For this review, take the finished solid that the model builds, in its own axes (mm). A direction names the side the tool comes from. Round coordinates to 2 decimals unless told otherwise and drop trailing zeros. Order: outer loops, then holes, each group sorted by start corner. A loop starts at its lowest first (then second) coordinate and runs counter-clockwise, first axis right, second up. Notation, with made-up numbers: (-25.5, 5) -> (-12.5, 5) arc R12 cw to (-12.5, 19) -> close; hole circle Ø7 at (24, 32.5). An arc over 180 degrees is marked (long way). Use a Markdown table: item, result. Add a question column.
1) Consider section D-D (x = 38). State the section outline as (y, z) points (3 decimals).
2) Consider section C-C (z = -15). State the section outline as (x, y) points.
3) Consider section A-A (z = -29). State the section outline as (x, y) points.
4) Consider section B-B (y = 17). State the section outline as (x, z) points (3 decimals), plus the area to 3 significant figures.
5) Machinability: for faces 1 (the face through (119.412, 9.536, -0.028)), 2 (the face through (-119, 4, -6.35)), 3 (the face through (-51.782, 9.658, -12.017)), which of the approach directions +Z, -Z, +X, -X, +Y, -Y give a long, thin tool a straight path to every point of the face, cutting with its end or side? Answer none if there is none.
6) Draft analysis for pull direction Z (two halves, no side actions). For faces 4 (the face through (1, 9, 0)), 5 (the face through (1, 0, -6)), 6 (the face through (-118.87, 10.03, -4.92)), 7 (the face through (5, 9, -9.525)), state which applies: pulls with the +Z half, pulls with the -Z half, needs draft (parallel to the pull), parting line crosses it, or undercut.
7) Clearance check with flat-ended pins moving along their axes: P1, Ø4, axis at y = 5, z = -19, coming from the -X side; P2, Ø8, axis at x = 121, y = 4, coming from the +Z side; P3, Ø1, axis at y = 16.5, z = -14.5, coming from the -X side. State where each tip first meets the part, or that it passes through.
8) Wall thickness on line 1 along X through (y, z) = (16, -1); line 2 along Y through (x, z) = (31.75, -6) (3 decimals); line 3 along X through (y, z) = (6.5, -20): over which ranges is each line inside the solid? List them lowest first. Write a range as [from, to].
```python
from build123d import *

# Parameters (mm, degrees)
BOSS_EXTRUDE1_DEPTH            = 19.05
FILLET1_R                      = 19.05
SKETCH2_R                      = 1.5
CUT_EXTRUDE1_DEPTH             = 129.572996096
BOSS_EXTRUDE2_REACH            = 132.835
BOSS_EXTRUDE2_END_RADIUS       = 25.4
CUT_EXTRUDE3_REACH             = 132.835
CUT_EXTRUDE3_DIRECTION_2_DEPTH = 131.83465787
CUT_EXTRUDE2_DEPTH             = 131.83465787
CUT_EXTRUDE2_DEPTH_BACK        = 131.83465787
FILLET2_R                      = 3.175
FILLET2_OF_MIRROR1_R           = 3.175
CUT_EXTRUDE4_DEPTH             = 131.834658007
CUT_EXTRUDE4_DEPTH_BACK        = 131.834658007


with BuildPart() as part:
    # Sketch1 → Boss-Extrude1 (new body)
    with BuildSketch(Plane(origin=(0, 0, 0), x_dir=(1, 0, 0), z_dir=(0, 1, 0))):
        with BuildLine():
            ThreePointArc((-54.639410761, 9.525), (-93.706612459, 35.233649778), (-124.46, 0))
            Line((-124.46, 0), (-114.3, 0))
            ThreePointArc((-114.3, 0), (-88.9, 25.4), (-63.5, 0))
            Line((-63.5, 0), (-53.34, 0))
            ThreePointArc((-53.34, 0), (-53.666350222, 4.806612459), (-54.639410761, 9.525))
        make_face()
        with BuildLine():
            Line((-53.34, 0), (0, 0))
            Line((0, 0), (0, 9.525))
            Line((0, 9.525), (-54.639410761, 9.525))
            ThreePointArc((-54.639410761, 9.525), (-53.666350222, 4.806612459), (-53.34, 0))
        make_face()
    boss_extrude1 = extrude(amount=BOSS_EXTRUDE1_DEPTH)

    # Fillet1
    fillet1_edges = [part.edges().sort_by_distance(p)[0] for p in [
        (-54.639410761, 9.525, -9.525),
    ]]
    fillet(fillet1_edges, radius=FILLET1_R)

    # Sketch2 → Cut-Extrude1 (cut, symmetric)
    with BuildSketch(Plane(origin=(0, 0, -9.525), x_dir=(-1, 0, 0), z_dir=(0, 0, -1))):
        with Locations((31.75, 9.525)):
            Circle(SKETCH2_R)
    cut_extrude1 = extrude(amount=CUT_EXTRUDE1_DEPTH, both=True, mode=Mode.SUBTRACT)

    # Boss-Extrude2: up to this cylinder (the profile starts outside it)
    boss_extrude2_end = Plane(origin=(-88.9, 11.6227675, 0), z_dir=(0, -1, 0)) * Cylinder(BOSS_EXTRUDE2_END_RADIUS, 323.358869, mode=Mode.PRIVATE)
    # Sketch3 → Boss-Extrude2 (add, up to the surface)
    with BuildSketch(Plane.ZY.offset(124.46), mode=Mode.PRIVATE) as boss_extrude2_sk1:
        Polygon((6.35, 19.05), (-6.35, 19.05), (-6.35, 12.065), (0, 9.525), (6.35, 9.525), align=None)
    boss_extrude2_tool1 = extrude(boss_extrude2_sk1.sketch, amount=-BOSS_EXTRUDE2_REACH, mode=Mode.PRIVATE) - boss_extrude2_end
    # Sketch3 → Boss-Extrude2 (add, up to the surface)
    with BuildSketch(Plane.ZY.offset(124.46), mode=Mode.PRIVATE) as boss_extrude2_sk2:
        Polygon((6.35, 6.985), (6.35, 9.525), (0, 9.525), align=None)
    boss_extrude2_tool2 = extrude(boss_extrude2_sk2.sketch, amount=-BOSS_EXTRUDE2_REACH, mode=Mode.PRIVATE) - boss_extrude2_end
    boss_extrude2 = boss_extrude2_tool1.solids().sort_by_distance((-124.46, 14.567202, 0.302381))[0] + boss_extrude2_tool2.solids().sort_by_distance((-124.46, 8.678333, 4.233333))[0]
    add(boss_extrude2)

    # Sketch3<3> → Cut-Extrude3 (cut, up to next)
    with BuildSketch(Plane.ZY.offset(124.46), mode=Mode.PRIVATE) as cut_extrude3_sk1:
        Polygon((-6.35, 0), (6.35, 0), (6.35, 6.985), (-6.35, 12.065), align=None)
    cut_extrude3_tool1 = extrude(cut_extrude3_sk1.sketch, amount=-CUT_EXTRUDE3_REACH, mode=Mode.PRIVATE) & part.part
    cut_extrude3 = cut_extrude3_tool1.solids().sort_by_distance((-124.46, 4.875389, -0.564444))[0]
    add(cut_extrude3, mode=Mode.SUBTRACT)

    # Sketch3<3> → Cut-Extrude3 direction 2 (cut)
    with BuildSketch(Plane.ZY.offset(124.46)):
        Polygon((-6.35, 0), (6.35, 0), (6.35, 6.985), (-6.35, 12.065), align=None)
    cut_extrude3_direction_2 = extrude(amount=CUT_EXTRUDE3_DIRECTION_2_DEPTH, mode=Mode.SUBTRACT)

    # Sketch4 → Cut-Extrude2 (cut, two sides: drawn at the far end of the back side and taken through both)
    with BuildSketch(Plane(origin=(0, 19.05, 0), x_dir=(1, 0, 0), z_dir=(0, 1, 0)).offset(-CUT_EXTRUDE2_DEPTH_BACK)):
        with BuildLine():
            Line((-124.46, -6.35), (-123.888442377, -6.35))
            ThreePointArc((-123.888442377, -6.35), (-124.316822351, -3.187835399), (-124.46, -2e-09))
            Line((-124.46, -2e-09), (-124.46, -6.35))
        make_face()
        with BuildLine():
            ThreePointArc((-124.46, -2e-09), (-124.316822351, 3.187835398), (-123.888442377, 6.35))
            Line((-123.888442377, 6.35), (-124.46, 6.35))
            Line((-124.46, 6.35), (-124.46, -2e-09))
        make_face()
    extrude(amount=CUT_EXTRUDE2_DEPTH + CUT_EXTRUDE2_DEPTH_BACK, mode=Mode.SUBTRACT)

    # Fillet2
    fillet2_edges = [part.edges().sort_by_distance(p)[0] for p in [
        (-118.690943313, 6.985, 6.35),
        (-118.690943313, 12.065, -6.35),
    ]]
    fillet(fillet2_edges, radius=FILLET2_R)

    # Mirror1: Boss-Extrude1, Cut-Extrude1, Boss-Extrude2, Cut-Extrude3, Cut-Extrude3 direction 2 across plane
    add(boss_extrude1.mirror(Plane(origin=(0, 19.05, 0), x_dir=(0, 0, 1), z_dir=(1, 0, 0))))
    add(cut_extrude1.mirror(Plane(origin=(0, 19.05, 0), x_dir=(0, 0, 1), z_dir=(1, 0, 0))), mode=Mode.SUBTRACT)
    add(boss_extrude2.mirror(Plane(origin=(0, 19.05, 0), x_dir=(0, 0, 1), z_dir=(1, 0, 0))))
    add(cut_extrude3.mirror(Plane(origin=(0, 19.05, 0), x_dir=(0, 0, 1), z_dir=(1, 0, 0))), mode=Mode.SUBTRACT)
    add(cut_extrude3_direction_2.mirror(Plane(origin=(0, 19.05, 0), x_dir=(0, 0, 1), z_dir=(1, 0, 0))), mode=Mode.SUBTRACT)

    # Fillet2 of Mirror1
    fillet2_of_mirror1_edges = [part.edges().sort_by_distance(p)[0] for p in [
        (118.690943313, 6.985, 6.35),
        (118.690943313, 12.065, -6.35),
    ]]
    fillet(fillet2_of_mirror1_edges, radius=FILLET2_OF_MIRROR1_R)

    # Sketch5 → Cut-Extrude4 (cut, two sides: drawn at the far end of the back side and taken through both)
    with BuildSketch(Plane(origin=(0, 19.05, 0), x_dir=(1, 0, 0), z_dir=(0, 1, 0)).offset(-CUT_EXTRUDE4_DEPTH_BACK)):
        with BuildLine():
            ThreePointArc((123.888442377, 6.35), (124.316822351, 3.187835399), (124.46, 0))
            Line((124.46, 0), (124.46, 6.35))
            Line((124.46, 6.35), (123.888442377, 6.35))
        make_face()
        with BuildLine():
            Line((124.46, -6.35), (124.46, 0))
            ThreePointArc((124.46, 0), (124.316822351, -3.187835399), (123.888442377, -6.35))
            Line((123.888442377, -6.35), (124.46, -6.35))
        make_face()
    extrude(amount=CUT_EXTRUDE4_DEPTH + CUT_EXTRUDE4_DEPTH_BACK, mode=Mode.SUBTRACT)


solid = part.part
```
Results list:
| question | item | result |
|---|---|---|
| 1 | outline | (0, -9.525) -> (19.05, -9.525) -> (19.05, 0) -> (0, 0) -> close |
| 2 | outline | (-121.14, 0) -> (-109.4, 0) -> (-109.4, 19.05) -> (-121.14, 19.05) -> close; (-68.4, 0) -> (-55.73, 0) -> (-55.73, 19.05) -> (-68.4, 19.05) -> close; (56.66, 0) -> (68.4, 0) -> (68.4, 19.05) -> (56.66, 19.05) -> close; (109.4, 0) -> (121.14, 0) -> (121.14, 19.05) -> (109.4, 19.05) -> close |
| 3 | outline | (-109.48, 0) -> (-68.32, 0) -> (-68.32, 19.05) -> (-109.48, 19.05) -> close; (68.32, 0) -> (109.48, 0) -> (109.48, 19.05) -> (68.32, 19.05) -> close |
| 4 | outline | (-123.888, 6.35) arc R35.56 ccw to (-58.597, -18.607) arc R19.05 cw to (-42.363, -9.525) -> (54.639, -9.525) arc R35.56 ccw to (123.888, 6.35) -> (113.493, 6.35) arc R25.4 cw (long way) to (63.5, 0) -> (-63.5, 0) arc R25.4 cw (long way) to (-113.493, 6.35) -> close |
| 4 | area | 3,120 mm2 |
| 5 | face 1 | +X, -Y |
| 5 | face 2 | +Z, -X, -Y |
| 5 | face 3 | -Z, +Y, -Y |
| 6 | face 4 | pulls with the +Z half |
| 6 | face 5 | needs draft |
| 6 | face 6 | undercut |
| 6 | face 7 | pulls with the -Z half |
| 7 | P1 | x = -120.13 |
| 7 | P2 | z = -6.29 |
| 7 | P3 | x = -121.59 |
| 8 | line 1 | [-124.45, -114.28], [-63.52, 63.52], [114.28, 124.45] |
| 8 | line 2 | [0, 8.025], [11.025, 19.05] |
| 8 | line 3 | [-118.3, -104.56], [-73.24, -59.5], [59.5, 73.24], [104.56, 118.3] |
